Autodesk Inventor part; units mm, degrees
ref_plane "YZ Plane" through (0, 0, 0) normal (1, 0, 0) x (0, 1, 0)
ref_plane "XZ Plane" through (0, 0, 0) normal (0, 1, 0) x (-1, 0, 0)
ref_plane "XY Plane" through (0, 0, 0) normal (0, 0, 1) x (1, 0, 0)
sketch "Skizze1" plane through (0, 0, 0) normal (0, 0, 1) x (1, 0, 0)
  line L0 (47.5, -10) -> (-47.5, -10)
  line L1 (-47.5, -10) -> (-47.5, 10)
  line L2 (-47.5, 10) -> (47.5, 10)
  line L3 (47.5, 10) -> (47.5, -10)
  line L4 (47.5, -10) -> (-47.5, 10) construction
  line L5 (-47.5, -10) -> (47.5, 10) construction
  circle A0 centre (-40.5, 0) radius 2.65
  circle A1 centre (9.5, 0) radius 2.65
  line L6 (-44.75, -2.4537) -> (-44.75, 2.4537)
  line L7 (-44.75, 2.4537) -> (-40.5, 4.9075)
  line L8 (-40.5, 4.9075) -> (-36.25, 2.4537)
  line L9 (-36.25, 2.4537) -> (-36.25, -2.4537)
  line L10 (-36.25, -2.4537) -> (-40.5, -4.9075)
  line L11 (-40.5, -4.9075) -> (-44.75, -2.4537)
  line L12 (5.25, -2.4537) -> (5.25, 2.4537)
  line L13 (5.25, 2.4537) -> (9.5, 4.9075)
  line L14 (9.5, 4.9075) -> (13.75, 2.4537)
  line L15 (13.75, 2.4537) -> (13.75, -2.4537)
  line L16 (13.75, -2.4537) -> (9.5, -4.9075)
  line L17 (9.5, -4.9075) -> (5.25, -2.4537)
  point P0 (0, 0)
  point P1 (0, 0)
  point P2 (0, 0)
  point P3 (-2.125, 0)
  point P4 (-2.125, 0)
  point P5 (-2.125, 0)
  dimension "d0" = 20
  dimension "d2" = 5.3
  dimension "d3" = 5.3
  dimension "d4" = 50
  dimension "d13" = 38
  dimension "d26" = 8.5
  dimension "d27" = 8.5
  dimension "d42" = 7
extrude "Extrusion1" add sketch "Skizze1" along normal blind 8.5 contours L0 L1 L2 L3 | L6 L7 L8 L9 L10 L11 | L12 L13 L14 L15 L16 L17
extrude "Extrusion2" cut sketch "Skizze1" along normal blind 6.5 contours A1 | L6 L7 L8 L9 L10 L11 | L12 L13 L14 L15 L16 L17
sketch "Skizze2" plane through (0, 0, 8.5) normal (0, 0, 1) x (1, 0, 0)
  line L0 (-47.5, -10) -> (47.5, -10)
  line L1 (47.5, -10) -> (47.5, 10)
  line L2 (47.5, 10) -> (-47.5, 10)
  line L3 (-47.5, 10) -> (-47.5, -10)
  line L4 (-47.5, 10) -> (-47.5, -10)
  line L5 (-47.5, 0) -> (47.5, 0) construction
  line L6 (47.5, -10) -> (47.5, 10)
  point P0 (0, 0)
  point P1 (-15.5, 0)
  point P2 (34.5, 0)
hole "Bohrung1" at (-15.5, 0, 8.5) at (34.5, 0, 8.5) direction (0, 0, -1) diameter 5.3 end through all counterbore diameter 10 counterbore depth 4
fillet "Rundung1" radius 5 2 edges at (-47.5, -10, 4.25) (-47.5, 10, 4.25)
sketch "Skizze3" plane through (0, 0, 8.5) normal (0, 0, 1) x (1, 0, 0)
  line L0 (39.5, 3) -> (29.5, 3)
  line L1 (29.5, 3) -> (29.5, -3)
  line L2 (29.5, -3) -> (39.5, -3)
  line L3 (39.5, -3) -> (39.5, 3)
  circle A0 centre (34.5, 0) radius 2.65
  line L4 (39.5, 3) -> (29.5, -3) construction
  line L5 (29.5, 3) -> (39.5, -3) construction
  circle A1 centre (-15.5, 0) radius 2.65
  line L6 (-10.5, 3) -> (-20.5, 3)
  line L7 (-20.5, 3) -> (-20.5, -3)
  line L8 (-20.5, -3) -> (-10.5, -3)
  line L9 (-10.5, -3) -> (-10.5, 3)
  line L10 (-10.5, 3) -> (-20.5, -3) construction
  line L11 (-20.5, 3) -> (-10.5, -3) construction
  point P0 (0, 0)
  dimension "d51" = 6
  dimension "d52" = 10
extrude "Extrusion4" cut sketch "Skizze3" against normal through all
equation "\"d3\" = d2"
equation "\"d27\" = d26"
properties part number "Door_Basis" material "ABS-Kunststoff"
The model under review builds one solid part; all positions refer to its coordinate system, in mm. A direction names the side the tool comes from. Coordinates: 2 decimals unless noted, no trailing zeros. Write each loop counter-clockwise with the first axis right and the second up, starting at its lowest first coordinate (ties: lowest second). Pieces come first, ordered by that corner, then holes.
1) To check wall thickness, follow probe 1 along X at (y, z) = (-1.5, 0.5); probe 2 along X at (y, z) = (-0.25, 7); probe 3 along Y at (x, z) = (-12, 1.5). State the ranges of each line that lie inside material, in increasing order.
2) Machinability: for faces 3 (the face through (34, -4, 4.5)), 4 (the face through (-38.405, 3.698, 3.204)), 5 (the face through (39.5, 0, 4)), which of the approach directions +Z, -Z, +X, -X, +Y, -Y give a long, thin tool a straight path to every point of the face, cutting with its end or side? Answer none if there is none.
3) We need section A-A on y = 0. State the section outline as (x, z) points, then the cut area to 3 significant figures.
4) We need section B-B on z = 2. State the section outline as (x, y) points.
5) Clearance check with a flat-ended pin moving along its axis: pin 1 Ø1.6 at (x, y) = (-16, 3.5) entering from +Z. State where the tip first meets the part, or that it passes through.
6) The part is to be moulded in two halves that separate along X. For faces 1 (the face through (-47.5, 0, 4)), 2 (the face through (7.6, -2.1, 6.5)), say which applies: pulls with the +X half, pulls with the -X half, needs draft (parallel to the pull), parting line crosses it, or undercut.
Answer list:
1. probe 1: x = -47.5 to -44.75, -36.25 to -20.5, -10.5 to 5.25, 13.75 to 29.5, 39.5 to 47.5
1. probe 2: x = -47.5 to -43.14, -37.86 to -20.5, -10.5 to 6.86, 12.14 to 29.5, 39.5 to 47.5
1. probe 3: y = -10 to -3, 3 to 10
2. face 3: +Z
2. face 4: -Z
2. face 5: +Z, -Z
3. outline: (-47.5, 0) - (-44.75, 0) - (-44.75, 6.5) - (-43.15, 6.5) - (-43.15, 8.5) - (-47.5, 8.5) - close; (-37.85, 6.5) - (-36.25, 6.5) - (-36.25, 0) - (-20.5, 0) - (-20.5, 8.5) - (-37.85, 8.5) - close; (-10.5, 0) - (5.25, 0) - (5.25, 6.5) - (6.85, 6.5) - (6.85, 8.5) - (-10.5, 8.5) - close; (12.15, 6.5) - (13.75, 6.5) - (13.75, 0) - (29.5, 0) - (29.5, 8.5) - (12.15, 8.5) - close; (39.5, 0) - (47.5, 0) - (47.5, 8.5) - (39.5, 8.5) - close
3. area: 506 mm2
4. outline: (-47.5, -5) arc R5 ccw to (-42.5, -10) - (47.5, -10) - (47.5, 10) - (-42.5, 10) arc R5 ccw to (-47.5, 5) - close; hole (-44.75, -2.45) - (-40.5, -4.91) - (-36.25, -2.45) - (-36.25, 2.45) - (-40.5, 4.91) - (-44.75, 2.45) - close; hole (-20.5, -3) - (-10.5, -3) - (-10.5, 3) - (-20.5, 3) - close; hole (5.25, -2.45) - (9.5, -4.91) - (13.75, -2.45) - (13.75, 2.45) - (9.5, 4.91) - (5.25, 2.45) - close; hole (29.5, -3) - (39.5, -3) - (39.5, 3) - (29.5, 3) - close
5. pin 1: stops at z = 4.5
6. face 1: pulls with the -X half
6. face 2: undercut
